Autodesk Inventor part; units mm, degrees
ref_plane "Work Plane2" through (0, 76.2, 0) normal (0, 1, 0) x (-1, 0, 0)
ref_plane "YZ Plane" through (0, 0, 0) normal (1, 0, 0) x (0, 1, 0)
ref_plane "XY Plane" through (0, 0, 0) normal (0, 0, 1) x (1, 0, 0)
sketch "Sketch1" plane through (0, 0, 0) normal (0, 0, 1) x (1, 0, 0)
  circle A0 centre (0, 0) radius 76.2
  dimension "d0" = 152.4
extrude "Extrusion1" add sketch "Sketch1" along normal mid plane 1828.8
ref_plane "Work Plane2" through (0, 76.2, 0) normal (0, 1, 0) x (-1, 0, 0)
sketch "Sketch4" plane through (0, 76.2, 0) normal (0, 1, 0) x (-1, 0, 0)
  line L0 (25.4, 635) -> (25.4, 584.2)
  line L1 (25.4, 584.2) -> (-25.4, 584.2)
  line L2 (-25.4, 584.2) -> (-25.4, 635)
  line L3 (-25.4, 635) -> (25.4, 635)
  line L4 (25.4, 635) -> (-25.4, 584.2) construction
  line L5 (25.4, 584.2) -> (-25.4, 635) construction
  line L6 (76.2, 914.4) -> (-76.2, 914.4)
  point P0 (0, 0)
  point P1 (0, 609.6)
  dimension "d17" = 50.8
  dimension "d19" = 304.8
extrude "Extrusion3" add sketch "Sketch4" against normal blind 25.4
mirror "Mirror1" about plane through (0, 0, 0) normal (0, 0, 1) of "Extrusion3"
sketch "Sketch5" plane through (0, 76.2, 0) normal (0, 1, 0) x (1, 0, 0)
  line L0 (76.2, 914.4) -> (-76.2, 914.4)
  line L1 (-76.2, -914.4) -> (76.2, -914.4)
  point P0 (0, 0)
  point P1 (0, -609.6)
  point P2 (0, 609.6)
  dimension "d22" = 304.8
  dimension "d23" = 304.8
hole "Hole2" at (0, 76.2, 609.6) at (0, 76.2, -609.6) direction (0, -1, 0) diameter 25.4 end through all
properties part number "CrossMember" material "Wood (Walnut)"
Design review of the part built by this model. Coordinates are the model's own, in mm. Round coordinates to 2 decimals unless told otherwise and drop trailing zeros. Write each loop counter-clockwise with the first axis right and the second up, starting at its lowest first coordinate (ties: lowest second). Pieces come first, ordered by that corner, then holes. Notation, with made-up numbers: (53.5, 54) -> (89.5, 54) arc R23 ccw to (89.5, 62) -> close; hole circle Ø4 at (45, 73.5). An arc over 180 degrees is marked (long way). One line per item, written item: value. Start each with the question number.
Q1. Add section A-A (y = -26.5). Give the boundary of the cut face in (x, z).
Q2. Add section B-B (z = 79.5). Give the boundary of the cut face in (x, y), then the cut area to 3 significant figures.
Q3. Add section D-D (x = 48). Give the boundary of the cut face in (y, z), then the cut area to 3 significant figures.
Q4. Add section C-C (x = -45.5). Give the boundary of the cut face in (y, z), then the cut area to 3 significant figures.
Q5. To check wall thickness, follow probe 1 along X at (y, z) = (-1, 610); probe 2 along Z at (x, y) = (0, 20.5); probe 3 along Z at (x, y) = (-10, -15.5). State the ranges of each line that lie inside material, in increasing order.
Q6. Insertion check: P1, Ø2, axis at x = 7.5, z = -668.5, coming from the +Y side; P2, Ø12, axis at y = 43, z = 637.5, coming from the -X side; P3, Ø5, axis at x = 52.5, z = 647, coming from the +Y side. Each pin has a flat end and moves straight along its axis. Give the tip position at first contact, or say it passes through.
Response:
1. outline: (-71.44, -914.4) -> (71.44, -914.4) -> (71.44, 914.4) -> (-71.44, 914.4) -> close; hole circle Ø25.4 at (0, -609.6); hole circle Ø25.4 at (0, 609.6)
2. outline: circle Ø152.4 at (0, 0)
2. area: 18,200 mm^2
3. outline: (-59.18, -914.4) -> (59.18, -914.4) -> (59.18, 914.4) -> (-59.18, 914.4) -> close
3. area: 216,000 mm^2
4. outline: (-61.12, -914.4) -> (61.12, -914.4) -> (61.12, 914.4) -> (-61.12, 914.4) -> close
4. area: 224,000 mm^2
5. probe 1: x = -76.19 to -12.69, 12.69 to 76.19
5. probe 2: z = -914.4 to -622.3, -596.9 to 596.9, 622.3 to 914.4
5. probe 3: z = -914.4 to -617.43, -601.77 to 601.77, 617.43 to 914.4
6. P1: stops at y = 75.92
6. P2: stops at x = -66.61
6. P3: stops at y = 57.5
